```python
from build123d import *

# Parameters (mm, degrees)
EXTRUDE_1_DEPTH          = 114
EXTRUDE_2_DEPTH          = 25
CUT_EXTRUDE_1_DEPTH      = 136.153981133
SKETCH_4_W               = 1
SKETCH_4_H               = 5
EXTRUDE_3_DEPTH          = 15
CUT_EXTRUDE_2_DEPTH      = 136.153981133
CUT_EXTRUDE_2_DEPTH_BACK = 136.153981133
SKETCH_5_W               = 9.764805651
SKETCH_5_H               = 37


with BuildPart() as part:
    # 草图1 → 凸台-拉伸1 (new body)
    with BuildSketch(Plane(origin=(0, 0, 0), x_dir=(1, 0, 0), z_dir=(0, 1, 0))):
        with BuildLine():
            Line((-50, 27.415384473), (-50, 24.5))
            ThreePointArc((-50, 24.5), (-48.267949192, 23.949489743), (-47.171572875, 22.5))
            Line((-47.171572875, 22.5), (-48.267949192, 22.5))
            ThreePointArc((-48.267949192, 22.5), (-52, 21.5), (-48.267949192, 20.5))
            Line((-48.267949192, 20.5), (-47.171572875, 20.5))
            ThreePointArc((-47.171572875, 20.5), (-51.060822526, 18.693818329), (-52.782628461, 22.62115068))
            add(Edge.make_bspline(
                [(-52.782628461, 22.62115068), (-77.601288898, 0), (-52.782628461, -22.62115068)],
                knots=[5.682111054, 5.682111054, 5.682111054, 6.884259561, 6.884259561, 6.884259561], degree=2, weights=[1, 0.82472857, 1]))
            ThreePointArc((-52.782628461, -22.62115068), (-51.060822526, -18.693818329), (-47.171572875, -20.5))
            Line((-47.171572875, -20.5), (-48.267949192, -20.5))
            ThreePointArc((-48.267949192, -20.5), (-52, -21.5), (-48.267949192, -22.5))
            Line((-48.267949192, -22.5), (-47.171572875, -22.5))
            ThreePointArc((-47.171572875, -22.5), (-48.267949192, -23.949489743), (-50, -24.5))
            Line((-50, -24.5), (-50, -27.415384473))
            add(Edge.make_bspline(
                [(-50, 27.415384473), (-87.12, 0), (-50, -27.415384473)],
                knots=[2.430387488, 2.430387488, 2.430387488, 3.85279782, 3.85279782, 3.85279782], degree=2, weights=[1, 0.757575758, 1]))
        make_face()
    extrude(amount=EXTRUDE_1_DEPTH)

    # 草图2 → 凸台-拉伸2 (add)
    with BuildSketch(Plane.XZ):
        with BuildLine():
            Line((-50, -24.968730444), (-50, -27.95708451))
            add(Edge.make_bspline(
                [(-50, 27.95708451), (-89.78, 0), (-50, -27.95708451)],
                knots=[5.554827697, 5.554827697, 5.554827697, 7.011542917, 7.011542917, 7.011542917], degree=2, weights=[1, 0.746268657, 1]))
            Line((-50, 27.95708451), (-50, 24.968730444))
            add(Edge.make_bspline(
                [(-50, 24.968730444), (-81.92, 0), (-50, -24.968730444)],
                knots=[5.609054801, 5.609054801, 5.609054801, 6.957315814, 6.957315814, 6.957315814], degree=2, weights=[1, 0.78125, 1]))
        make_face()
    extrude(amount=-EXTRUDE_2_DEPTH)

    # 草图3 → 切除-拉伸1 (cut, through all)
    with BuildSketch(Plane(origin=(0, 0, 0), x_dir=(0, 0, -1), z_dir=(1, 0, 0))):
        with BuildLine():
            Line((3, 114), (-3, 114))
            Line((-3, 114), (-3, 102))
            ThreePointArc((-3, 102), (0, 99), (3, 102))
            Line((3, 102), (3, 114))
        make_face()
    extrude(amount=-CUT_EXTRUDE_1_DEPTH, mode=Mode.SUBTRACT)

    # 草图4 → 凸台-拉伸3 (add)
    with BuildSketch(Plane(origin=(0, 114, 0), x_dir=(1, 0, 0), z_dir=(0, 1, 0))):
        with Locations((-63.319746161, 5.5)):
            Rectangle(SKETCH_4_W, SKETCH_4_H)
        with Locations((-63.319746161, -5.5)):
            Rectangle(SKETCH_4_W, SKETCH_4_H)
    extrude(amount=-EXTRUDE_3_DEPTH)

    # 草图5 → 切除-拉伸2 (cut, two sides: drawn at the far end of the back side and taken through both)
    with BuildSketch(Plane.XY.offset(-CUT_EXTRUDE_2_DEPTH_BACK)):
        with Locations((-45.117597175, 85.5)):
            Rectangle(SKETCH_5_W, SKETCH_5_H)
        with Locations((-45.117597175, 28.5)):
            Rectangle(SKETCH_5_W, SKETCH_5_H)
    extrude(amount=CUT_EXTRUDE_2_DEPTH + CUT_EXTRUDE_2_DEPTH_BACK, mode=Mode.SUBTRACT)


solid = part.part
```
Here's how the part is built. I have some questions about the finished solid (model axes, mm). A direction names the side the tool comes from. Coordinates: 2 decimals unless noted, no trailing zeros. Use a Markdown table: item, result. Add a question column.
(1) For faces 4 (the flat face through (-62.82, 107, -5)), 5 (the cylindrical face through (-52, 56.2, 21.43)), 6 (the cylindrical face through (-48.2, 56.9, 23.9)), 7 (the flat face through (-65, 25, 8)), 8 (the flat face through (-49, 10, 19)), which set-ups out of +Z, -Z, +X, -X, +Y, -Y let a thin tool reach every point of the face, with its end or its side?
(2) We'd pull the mould along X, two halves only. Please class faces 1 (the flat face through (-49, 67, 19)), 2 (the cylindrical face through (-52, 56.2, -21.57)), 3 (the flat face through (-50, 56, 26)): +X half, -X half, draft (parallel to the pull), parting line (faces both ways), or undercut.
(3) I'm going to push flat-ended pins straight in: P1, Ø4, axis at y = 52.5, z = -7.5, coming from the +X side; P2, Ø0.6, axis at x = -48.5, z = 19.5, coming from the -Y side; P3, Ø5, axis at x = -59, y = 99.5, coming from the +Z side; P4, Ø3.5, axis at y = 77.5, z = -25, coming from the +X side. Where does each tip first touch, or does it pass through?
(4) Please list where these lines run through material, in increasing order: line 1 (Z direction, x = -48.25, y = 56); line 2 (Z direction, x = -57.25, y = 55.5); line 3 (Z direction, x = -54.5, y = 38.5).
Outcome:
| question | item | result |
|---|---|---|
| 1 | face 4 | +X, +Y, -Y |
| 1 | face 5 | +Y, -Y |
| 1 | face 6 | +Z, +X, +Y, -Y |
| 1 | face 7 | -X, +Y |
| 1 | face 8 | +Z, -Z, +X |
| 2 | face 1 | draft |
| 2 | face 2 | undercut |
| 2 | face 3 | +X half |
| 3 | P1 | stops at x = -62.17 |
| 3 | P2 | stops at y = 0 |
| 3 | P3 | stops at z = 21.71 |
| 3 | P4 | stops at x = -50 |
| 4 | line 1 | z = -23.94 to -22.5, -20.5 to -19.06, 19.06 to 20.5, 22.5 to 23.94 |
| 4 | line 2 | z = -20.9 to -17.88, 17.88 to 20.9 |
| 4 | line 3 | z = -23.69 to -20.97, 20.97 to 23.69 |
